CAD build for the part. Positions are in the model's coordinates, mm. A direction names the side the tool comes from. Round coordinates to 2 decimals unless told otherwise and drop trailing zeros. Loops run counter-clockwise (first coordinate to the right, second up) from the corner with the lowest first, then second, coordinate; pieces in that order, holes last. Notation, with made-up numbers: M -15.5,-22.75 L 20.5,-22.75 A34 ccw 20.5,11.25 Z; hole C 42,69.5 d7. An arc over 180 degrees is marked long. Use a Markdown table: item, result. Add a question column.
(1) Wall check: L1, parallel to Y at x = -37.5, z = -77.25; L2, parallel to Z at x = 49.5, y = 118; L3, parallel to Y at x = 49.5, z = -79.6. Give the ranges that are in metal, low to high.
(2) Band-saw the part on A-A, the plane x = -67. Write the cut outline in (y, z), and give its area (3 significant figures).
(3) Which spindle directions (+Z, -Z, +X, -X, +Y, -Y) get a long thin tool onto all of the face, cutting with end or side? Do faces 4 (the face through (-0.682, 87.368, -73.535)), 5 (the face through (-67.4, -18.16, -67.62)), 6 (the face through (-2, 92, -74)), 7 (the face through (2, 7, -74)), 8 (the face through (37.43, 110.98, -78.03)). Say none if no direction does.
(4) Flat gauge pins, fed straight in: P1, Ø24.5, axis at x = -2.5, y = 31, coming from the +Z side; P2, Ø4, axis at x = -22.5, z = -72.5, coming from the +Y side; P3, Ø2, axis at x = -11.5, z = -71, coming from the -Y side. Where does each tip first touch, or does it go through?
(5) Band-saw the part on C-C, the plane x = -31. Write the cut outline in (y, z), and give its area (3 significant figures).
(6) Two-plate mould, pull along Y, no slides. Class faces 1 (the face through (59.058, 127.934, -66.417)), 2 (the face through (-61.668, -26.678, -62.017)), 3 (the face through (6.231, -4.175, -77.972)): released by +Y, released by -Y, zero draft, split by the parting line, or undercut.
(7) Band-saw the part on B-B, the plane y = 81.5. Write the cut outline in (x, z).
from build123d import *

# Parameters (mm, degrees)
SKETCH2_R           = 0.5
SKETCH2_R_2         = 0.49999999999999917
SKETCH2_R_3         = 0.5000000000000001
BOSS_EXTRUDE1_DEPTH = 4
CHAMFER1_SIZE       = 3
BOSS_EXTRUDE2_DEPTH = 4
FILLET1_R           = 10
BOSS_EXTRUDE4_DEPTH = 5
CHAMFER2_SIZE       = 5
BOSS_EXTRUDE5_DEPTH = 12
CHAMFER3_SIZE       = 4
SKETCH7_R           = 1.9999999999999967
CUT_EXTRUDE1_DEPTH  = 197.57038973194156
SKETCH8_R           = 1.7500000000000013
SKETCH8_R_2         = 1.7500000000000038
SKETCH8_R_3         = 1.7499999999999993
CUT_EXTRUDE2_DEPTH  = 10
CUT_EXTRUDE3_START  = -4
SKETCH9_R           = 2.5000000000000027
SKETCH9_R_2         = 2.5000000000000018
SKETCH9_R_3         = 2.5
CUT_EXTRUDE3_DEPTH  = 10
BOSS_EXTRUDE6_DEPTH = 4


with BuildPart() as part:
    # Sketch2 → Boss-Extrude1 (new body)
    with BuildSketch(Plane(origin=(-1.25e-15, -1.7e-16, -75.99999999999999), x_dir=(-1, 0, 2e-17), z_dir=(-2e-17, 0, -1))):
        with BuildLine():
            Line((-7.5, 42.00000000000002), (-7.5, -2.45e-15))
            ThreePointArc((-7.5, -2.45e-15), (1e-16, -7.5), (7.5, -1.8e-15))
            Line((7.5, 1.12e-15), (7.5, 41.999999999999964))
            Line((7.5, 41.999999999999964), (49.50000000000001, 41.99999999999978))
            ThreePointArc((49.50000000000001, 41.99999999999978), (57.0000000000001, 49.49999999999975), (49.50000000000007, 56.99999999999978))
            Line((49.500000000000064, 56.99999999999979), (7.5, 56.99999999999995))
            Line((7.5, 56.99999999999995), (7.499999999999976, 99.00000000000001))
            ThreePointArc((7.499999999999975, 99.00000000000001), (-2.319e-14, 106.5), (-7.500000000000025, 99.00000000000001))
            Line((-7.500000000000024, 99.00000000000001), (-7.500000000000015, 57.000000000000014))
            Line((-7.5, 57.000000000000014), (-49.49999999999994, 57.00000000000019))
            ThreePointArc((-49.49999999999994, 57.00000000000019), (-57.000000000000064, 49.50000000000023), (-49.49999999999999, 42.000000000000206))
            Line((-49.49999999999999, 42.0000000000002), (-7.5, 42.00000000000002))
        make_face()
        Circle(SKETCH2_R, mode=Mode.SUBTRACT)
        with Locations((49.5, 49.49999999999988)):
            Circle(SKETCH2_R_2, mode=Mode.SUBTRACT)
        with Locations((-49.5, 49.50000000000013)):
            Circle(SKETCH2_R_2, mode=Mode.SUBTRACT)
        with Locations((-2.352e-14, 99)):
            Circle(SKETCH2_R_3, mode=Mode.SUBTRACT)
    extrude(amount=BOSS_EXTRUDE1_DEPTH)

    # Chamfer1
    chamfer1_edges = [part.edges().sort_by_distance(p)[0] for p in [
        (0.49999999999999867, -1.1e-16, -75.99999999999999),
        (-49, 49.49999999999988, -75.99999999999999),
        (0.5000000000000224, 99, -75.99999999999999),
        (50, 49.50000000000013, -75.99999999999999),
    ]]
    chamfer(chamfer1_edges, length=CHAMFER1_SIZE)

    # Sketch3 → Boss-Extrude2 (add)
    with BuildSketch(Plane(origin=(0, 0, -79.99999999999999), x_dir=(-1, 0, 0), z_dir=(0, 0, -1))):
        Polygon((56.48320781823236, 52.235837818178865), (80.96372644585969, -10.250523010263308), (70.35712472806149, -20.85712472806152), (65.40737725975566, -15.907377259755682), (70.46028645315, -10.854468066361337), (49.7516366918705, 42.004222590330855), align=None)
    extrude(amount=-BOSS_EXTRUDE2_DEPTH)

    # Fillet1
    fillet1_edges = [part.edges().sort_by_distance(p)[0] for p in [
        (-49.7516366918705, 42.004222590330855, -77.99999999999999),
    ]]
    fillet(fillet1_edges, radius=FILLET1_R)

    # Sketch5 → Boss-Extrude4 (add)
    with BuildSketch(Plane.XY.offset(-75.99999999999999)):
        with BuildLine():
            Line((0, 49.49999999999989), (-2.0000000000000018, 51.49999999999989))
            Line((-2.0000000000000018, 51.49999999999989), (-46.62771867673098, 51.499999999999886))
            ThreePointArc((-46.62771867673098, 51.499999999999886), (-45.999999999999986, 49.499999999999886), (-46.627718676730964, 47.499999999999886))
            Line((-46.627718676730964, 47.499999999999886), (-1.9999999999999982, 47.499999999999886))
            Line((-1.9999999999999982, 47.499999999999886), (0, 49.49999999999989))
        make_face()
        with BuildLine():
            Line((-54.33302242729803, 49.49999999999989), (-76.5772611619678, -7.2782712887445))
            Line((-76.5772611619678, -7.2782712887445), (-80.25661966467315, -10.957629791449861))
            Line((-80.25661966467315, -10.957629791449861), (-78.64868432735105, -12.56556512877197))
            Line((-78.64868432735105, -12.56556512877197), (-70.35712472806149, -20.85712472806152))
            Line((-70.35712472806149, -20.85712472806152), (-67.5286976033153, -18.028697603315333))
            Line((-67.5286976033153, -18.028697603315333), (-73.96959982780758, -11.587795378823028))
            Line((-73.96959982780758, -11.587795378823028), (-51.229176548510004, 46.45698365694761))
            ThreePointArc((-51.229176548510004, 46.45698365694761), (-52.525071728057476, 47.73961906392169), (-53.00000000000002, 49.4999999999999))
            Line((-53.00000000000002, 49.4999999999999), (-54.33302242729803, 49.49999999999989))
        make_face()
    extrude(amount=BOSS_EXTRUDE4_DEPTH)

    # Chamfer2
    chamfer2_edges = [part.edges().sort_by_distance(p)[0] for p in [
        (-45.999999999999986, 49.499999999999886, -70.99999999999999),
        (-52.525071728057476, 47.73961906392169, -70.99999999999999),
    ]]
    chamfer(chamfer2_edges, length=CHAMFER2_SIZE - 0.0001)  # a hair under: the kernel refuses the full size

    # Mirror2: part across plane


with BuildPart() as part_1:
    add(part.part)
    add(part.part.mirror(Plane(origin=(-70.35712472806149, -20.85712472806152, 3.478146182439232), x_dir=(0, 0, 1), z_dir=(0.7071067811865482, -0.7071067811865468, 0))))

    # Sketch6 → Boss-Extrude5 (add)
    with BuildSketch(Plane.XY.offset(-70.99999999999999)):
        Polygon((-80.25661966467315, -10.957629791449861), (-60.45762979144981, -30.75661966467317), (-58.00107255414479, -27.5563226524858), (-77.05632265248579, -8.501072554144805), align=None)
    extrude(amount=BOSS_EXTRUDE5_DEPTH)

    # Chamfer3
    chamfer3_edges = [part_1.edges().sort_by_distance(p)[0] for p in [
        (-59.54443396648389, -26.012961240146698, -70.99999999999999),
        (-75.51296124014668, -10.044433966483911, -70.99999999999999),
    ]]
    chamfer(chamfer3_edges, length=CHAMFER3_SIZE)

    # Sketch7 → Cut-Extrude1 (cut, through all)
    with BuildSketch(Plane(origin=(-42.77869760331542, -42.7786976033153, 0), x_dir=(0, 0, -1), z_dir=(0.7071067811865475, 0.7071067811865477, 0))):
        with Locations(Location((63.99999999999996, 45.00178566873401, 0), (0, 0, 90))):
            Circle(SKETCH7_R)
        with Locations(Location((63.99999999999996, 25.001785668734005, 0), (0, 0, 90))):
            Circle(SKETCH7_R)
    extrude(amount=-CUT_EXTRUDE1_DEPTH, mode=Mode.SUBTRACT)

    # Mirror3: part across plane


with BuildPart() as part_2:
    add(part_1.part)
    add(part_1.part.mirror(Plane(origin=(0, 49.49999999999989, -70.99999999999999), x_dir=(0, 0, 1), z_dir=(-0.7071067811865476, -0.7071067811865476, 0))))

    # Sketch8 → Cut-Extrude2 (cut)
    with BuildSketch(Plane(origin=(0, 0, -79.99999999999999), x_dir=(-1, 0, 0), z_dir=(0, 0, -1))):
        with Locations((3.1819805153394918, 87.33021279348041)):
            Circle(SKETCH8_R)
        with Locations((37.83021279348029, 52.68198051533957)):
            Circle(SKETCH8_R_2)
        with Locations((-3.1819805153395033, 11.669787206519844)):
            Circle(SKETCH8_R_3)
        with Locations((-37.83021279348031, 46.31801948466069)):
            Circle(SKETCH8_R_2)
    extrude(amount=-CUT_EXTRUDE2_DEPTH, mode=Mode.SUBTRACT)

    # Sketch9 → Cut-Extrude3 (cut)
    with BuildSketch(Plane(origin=(0, 0, -79.99999999999999), x_dir=(-1, 0, 0), z_dir=(0, 0, -1)).offset(CUT_EXTRUDE3_START)):
        with Locations((-37.83021279348031, 46.31801948466069)):
            Circle(SKETCH9_R)
        with Locations((3.1819805153394918, 87.33021279348041)):
            Circle(SKETCH9_R_2)
        with Locations((37.83021279348029, 52.68198051533957)):
            Circle(SKETCH9_R)
        with Locations((-3.1819805153395038, 11.669787206519844)):
            Circle(SKETCH9_R_3)
    extrude(amount=-CUT_EXTRUDE3_DEPTH, mode=Mode.SUBTRACT)

    # Sketch10 → Boss-Extrude6 (add)
    with BuildSketch(Plane(origin=(0, 0, -79.99999999999999), x_dir=(-1, 0, 0), z_dir=(0, 0, -1))):
        Polygon((-7.499999999999999, 71.14213562373105), (21.642135623731086, 41.99999999999998), (7.5000000000001386, 27.857864376269028), (-21.642135623730947, 57.0000000000001), align=None)
    extrude(amount=-BOSS_EXTRUDE6_DEPTH)


solid = part_2.part
Return value:
| question | item | result |
|---|---|---|
| 1 | L1 | -22.75 to -12.01, 42 to 50.96, 54.4 to 57 |
| 1 | L2 | -80 to -76 |
| 1 | L3 | 42 to 49, 50 to 59.46, 115.71 to 126.45 |
| 2 | outline | M -24.21,-80 L -14.31,-80 L -14.31,-76 L -18.56,-76 L -18.56,-59 L -24.21,-59 Z; M -2.02,-80 L 25.39,-80 L 25.39,-76 L 17.17,-76 L 17.17,-71 L 6.2,-71 L 6.2,-76 L -2.02,-76 Z |
| 2 | area | 300 mm^2 |
| 3 | face 4 | +Z, -X |
| 3 | face 5 | +Z |
| 3 | face 6 | +Z, -X, +Y |
| 3 | face 7 | +Z, +X, -Y |
| 3 | face 8 | +Z, -Z |
| 4 | P1 | z = -71 |
| 4 | P2 | y = 51.5 |
| 4 | P3 | y = -9.73 |
| 5 | outline | M -20.2,-80 L -9.46,-80 L -9.46,-76 L -12.68,-76 L -12.68,-71 L -16.98,-71 L -16.98,-76 L -20.2,-76 Z; M 42,-80 L 57,-80 L 57,-76 L 51.5,-76 L 51.5,-71 L 47.5,-71 L 47.5,-76 L 42,-76 Z |
| 5 | area | 144 mm^2 |
| 6 | face 1 | released by +Y |
| 6 | face 2 | undercut |
| 6 | face 3 | released by -Y |
| 7 | outline | M -7.5,-80 L 7.5,-80 L 7.5,-76 L 2,-76 L 2,-71 L -2,-71 L -2,-76 L -7.5,-76 Z; M 59.35,-80 L 70.09,-80 L 70.09,-76 L 66.87,-76 L 66.87,-71 L 62.57,-71 L 62.57,-76 L 59.35,-76 Z |
